Verification items for the finished model (mm, model axes). Round coordinates to 2 decimals unless told otherwise and drop trailing zeros. Order: outer loops, then holes, each group sorted by start corner. A loop starts at its lowest first (then second) coordinate and runs counter-clockwise, first axis right, second up. Notation, with made-up numbers: (52, 27.5) -> (85, 27.5) arc R26 cw to (85, 41.5) -> close; hole circle Ø8 at (-14, 58). An arc over 180 degrees is marked (long way). Put each result on its own line as item: value.
from build123d import *

# Parameters (mm, degrees)
EXTRUDE_1_DEPTH    = 4
SKETCH_2_W         = 20
SKETCH_2_H         = 4
EXTRUDE_2_DEPTH    = 5.5
SKETCH1_W          = 4.4
SKETCH1_H          = 17.190587951
CUT_EXTRUDE1_DEPTH = 10
LPATTERN1_COUNT    = 2
LPATTERN1_PITCH    = 25
SKETCH3_W          = 11.685912807
SKETCH3_H          = 13.236550351
CUT_EXTRUDE3_DEPTH = 10
SKETCH2_W          = 16.35313114
SKETCH2_H          = 2.289354212
SKETCH2_W_2        = 12.3172739
SKETCH2_H_2        = 5.182620656
CUT_EXTRUDE4_DEPTH = 10
SKETCH4_W          = 4.4
SKETCH4_H          = 12.896988848
CUT_EXTRUDE5_DEPTH = 10
LPATTERN2_COUNT    = 2
LPATTERN2_PITCH    = 25


with BuildPart() as part:
    # Эскиз1 → Бобышка-Вытянуть1 (new body)
    with BuildSketch(Plane(origin=(0, 0, 0), x_dir=(1, 0, 0), z_dir=(0, 1, 0))):
        Polygon((-14.85, 14.498494424), (5.95, 14.498494424), (5.95, 11.498494424), (10.15, 11.498494424), (10.15, 14.498494424), (124.5, 14.498494424), (124.5, -14.498494424), (-124.5, -14.498494424), (-124.5, 14.498494424), (-19.05, 14.498494424), (-19.05, 11.498494424), (-14.85, 11.498494424), align=None)
    extrude(amount=EXTRUDE_1_DEPTH)

    # Эскиз2 → Бобышка-Вытянуть2 (add)
    with BuildSketch(Plane(origin=(124.5, 0, 0), x_dir=(0, 0, -1), z_dir=(1, 0, 0))):
        with Locations((0, 2)):
            Rectangle(SKETCH_2_W, SKETCH_2_H)
    extrude_2 = extrude(amount=EXTRUDE_2_DEPTH)

    # Mirror1: Бобышка-Вытянуть2 across plane
    add(extrude_2.mirror(Plane(origin=(0, 0, 0), x_dir=(0, 0, 1), z_dir=(1, 0, 0))))

    # Sketch1 → Cut-Extrude1 (cut)
    with BuildSketch(Plane(origin=(0, 4, 0), x_dir=(1, 0, 0), z_dir=(0, 1, 0))):
        with Locations((-67.763838692, 5.903200448)):
            Rectangle(SKETCH1_W, SKETCH1_H)
    cut_extrude1 = extrude(amount=-CUT_EXTRUDE1_DEPTH, mode=Mode.SUBTRACT)

    # LPattern1: Cut-Extrude1 ×2
    with Locations(*[(-i * LPATTERN1_PITCH, 0, 0) for i in range(1, LPATTERN1_COUNT)]):
        add(cut_extrude1, mode=Mode.SUBTRACT)

    # Sketch3 → Cut-Extrude3 (cut)
    with BuildSketch(Plane(origin=(0, 0, 0), x_dir=(1, 0, 0), z_dir=(0, 1, 0))):
        with Locations((-31.80775481, 4.169260767)):
            Rectangle(SKETCH3_W, SKETCH3_H)
    extrude(amount=CUT_EXTRUDE3_DEPTH, mode=Mode.SUBTRACT)

    # Sketch2 → Cut-Extrude4 (cut)
    with BuildSketch(Plane.XZ):
        with Locations((-15.10817653, 3.144359058)):
            Rectangle(SKETCH2_W, SKETCH2_H)
        with Locations((-15.029613665, 6.880346492)):
            Rectangle(SKETCH2_W_2, SKETCH2_H_2)
    extrude(amount=-CUT_EXTRUDE4_DEPTH, mode=Mode.SUBTRACT)

    # Sketch4 → Cut-Extrude5 (cut)
    with BuildSketch(Plane(origin=(0, 4, 0), x_dir=(1, 0, 0), z_dir=(0, 1, 0))):
        with Locations((72.185759894, -8.05)):
            Rectangle(SKETCH4_W, SKETCH4_H)
    cut_extrude5 = extrude(amount=-CUT_EXTRUDE5_DEPTH, mode=Mode.SUBTRACT)

    # LPattern2: Cut-Extrude5 ×2
    with Locations(*[(i * LPATTERN2_PITCH, 0, 0) for i in range(1, LPATTERN2_COUNT)]):
        add(cut_extrude5, mode=Mode.SUBTRACT)


solid = part.part
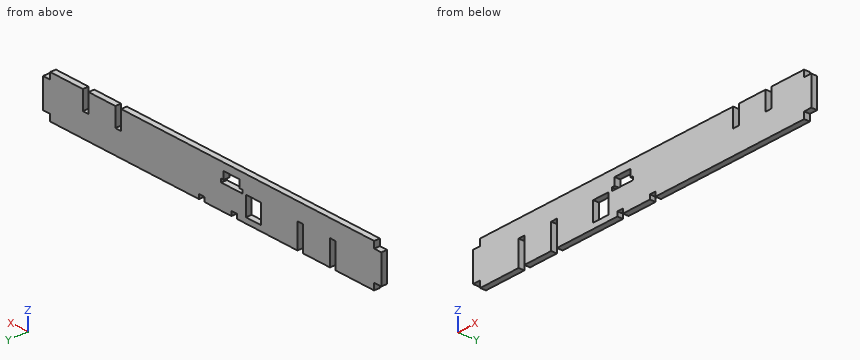
Item 1: Section check A-A on z = -2. Record the boundary of the cut face in (x, y), then the cut area to 3 significant figures.
Check sheet entries:
outline: (-130, 0) -> (-94.96, 0) -> (-94.96, 4) -> (-130, 4) -> close; (-90.56, 0) -> (-69.96, 0) -> (-69.96, 4) -> (-90.56, 4) -> close; (-65.56, 0) -> (-37.65, 0) -> (-37.65, 4) -> (-65.56, 4) -> close; (-25.96, 0) -> (130, 0) -> (130, 4) -> (-25.96, 4) -> close
area: 958 mm^2
Item 2: Gauge pin test, flat ends, axial feed: pin 1 Ø1.2 at (x, y) = (97, 2.5) entering from +Z; pin 2 Ø0.9 at (y, z) = (3, -13.5) entering from -X; pin 3 Ø1.2 at (x, y) = (-127.5, 1.5) entering from +Z. Record the tip position at first contact, or that the pin passes through.
Check sheet entries:
pin 1: stops at z = 1.6
pin 2: stops at x = -124.5
pin 3: stops at z = 10
Item 3: Material ranges on L1, parallel to X at y = 0.95, z = 11.25; L2, parallel to X at y = 3.05, z = -13; L3, parallel to X at y = 0.7, z = 5.5, recorded low to high. Write a range as [from, to].
Check sheet entries:
L1: x = [-124.5, 69.99], [74.39, 94.99], [99.39, 124.5]
L2: x = [-124.5, -94.96], [-90.56, -69.96], [-65.56, -19.05], [-14.85, 5.95], [10.15, 124.5]
L3: x = [-130, -21.19], [-8.87, 69.99], [74.39, 94.99], [99.39, 130]
Item 4: Section check B-B on y = 2. State how many separate pieces and enclosed holes the cut face has, then the cut area to 3 significant figures.
Check sheet entries:
separate pieces: 1
enclosed holes: 2
area: 6,890 mm^2
